```python
from build123d import *

# Parameters (mm, degrees)
BOSS_EXTRUDE1_DEPTH      = 5
BOSS_EXTRUDE2_DEPTH      = 1
BOSS_EXTRUDE2_DEPTH_BACK = 1
SKETCH4_W                = 2
SKETCH4_H                = 1
SKETCH4_W_2              = 17
SKETCH4_H_2              = 2
SKETCH5_R                = 0.75
BOSS_EXTRUDE3_DEPTH      = 5
FILLET1_R                = 4


with BuildPart() as part:
    # Sketch1 → Boss-Extrude1 (new body)
    with BuildSketch(Plane(origin=(0, 0, 0), x_dir=(1, 0, 0), z_dir=(0, 1, 0))):
        with BuildLine():
            Line((0, 14.4), (25, 14.4))
            ThreePointArc((25, 14.4), (39.4, 0), (25, -14.4))
            Line((25, -14.4), (0, -14.4))
            ThreePointArc((0, -14.4), (-14.4, 0), (0, 14.4))
        make_face()
        with BuildLine():
            Line((0, 12.4), (25, 12.4))
            ThreePointArc((25, 12.4), (37.4, 0), (25, -12.4))
            Line((25, -12.4), (0, -12.4))
            ThreePointArc((0, -12.4), (-12.4, 0), (0, 12.4))
        make_face(mode=Mode.SUBTRACT)
    extrude(amount=BOSS_EXTRUDE1_DEPTH)

    # Sketch4 → Boss-Extrude2 (add, two sides: drawn at the far end of the back side and taken through both)
    with BuildSketch(Plane.XY.offset(-BOSS_EXTRUDE2_DEPTH_BACK)):
        Polygon((-31.4, 12), (-29.4, 12), (-29.4, 13), (-32.4, 13), (-32.4, 11), (-31.4, 11), align=None)
        with Locations((-30.4, 11.5)):
            Rectangle(SKETCH4_W, SKETCH4_H)
        Polygon((-29.4, 3), (-29.4, 5), (-29.4, 11), (-31.4, 11), (-31.4, 3), align=None)
        with Locations((-20.9, 4)):
            Rectangle(SKETCH4_W_2, SKETCH4_H_2)
    extrude(amount=BOSS_EXTRUDE2_DEPTH + BOSS_EXTRUDE2_DEPTH_BACK)

    # Sketch5 → Boss-Extrude3 (add)
    with BuildSketch(Plane.ZY.offset(32.4)):
        with Locations((0, 12)):
            Circle(SKETCH5_R)
    extrude(amount=BOSS_EXTRUDE3_DEPTH)

    # Fillet1
    # the kernel refuses this fillet: 4 mm, written as the material it adds along each edge
    with BuildSketch(Plane(origin=(-14.365235814, 5, -1), x_dir=(0.17149804582148126, 0, -0.9851844600273663), z_dir=(0, -1, 0))) as fillet1_piece_1:
        with BuildLine():
            CenterArc((3.367524545, -3.978862537), FILLET1_R, 95.892851455, 74.232218513)
            Line((-0.573213295, -3.292870354), (-0.652028052, -3.27915051))
            Line((-0.652028052, -3.27915051), (-0.078814757, 0.013719844))
            Line((-0.078814757, 0.013719844), (0.008213474, 0.079577251))
            ThreePointArc((0.008213474, 0.079577251), (1.47842541, 0.003905135), (2.948637345, 0.079577251))
            Line((2.948637345, 0.079577251), (2.95685082, 0))
        make_face()
    extrude(amount=2)
    with BuildSketch(Plane(origin=(-14.365235814, 5, 1), x_dir=(0.17149804582148112, 0, 0.9851844600273663), z_dir=(0, -1, 0))) as fillet1_piece_2:
        with BuildLine():
            CenterArc((3.367524545, 3.978862537), FILLET1_R, 189.874930032, 74.232218513)
            Line((-0.573213295, 3.292870354), (-0.652028052, 3.27915051))
            Line((-0.652028052, 3.27915051), (-0.078814757, -0.013719844))
            Line((-0.078814757, -0.013719844), (0.008213474, -0.079577251))
            ThreePointArc((0.008213474, -0.079577251), (1.47842541, -0.003905135), (2.948637345, -0.079577251))
            Line((2.948637345, -0.079577251), (2.95685082, 0))
        make_face()
    extrude(amount=2)
    with BuildSketch(Plane(origin=(0, 3, 0), x_dir=(-0.7371891614816782, 0, 0.6756864214959037), z_dir=(0.6756864214959037, 0, 0.7371891614816782))) as fillet1_piece_3_section:
        with BuildLine():
            CenterArc((18.272983346, 4), FILLET1_R, 194.477512186, 75.522487814)
            Line((18.272983346, 0), (18.272983346, -0.08))
            Line((18.272983346, -0.08), (14.4, -0.08))
            Line((14.4, -0.08), (14.32, 0))
            ThreePointArc((14.32, 0), (14.32, 1.5), (14.322540333, 2.98))
            Line((14.322540333, 2.98), (14.4, 3))
        make_face()
    fillet1_piece_3 = revolve(axis=Axis((0, 3, 0), (0, -1, 0)), revolution_arc=85.014954966, mode=Mode.PRIVATE)
    fillet1_piece_3 = split(fillet1_piece_3, bisect_by=Plane(origin=(-15.301586286, 2.241601932, -1), z_dir=(0, 0, 1)), keep=Keep.TOP, mode=Mode.PRIVATE)
    fillet1_piece_3 = split(fillet1_piece_3, bisect_by=Plane(origin=(-15.301586286, 2.241601932, 1), z_dir=(0, 0, -1)), keep=Keep.TOP, mode=Mode.PRIVATE)
    add(fillet1_piece_3)
    with BuildSketch(Plane(origin=(-29.4, 5, 1), x_dir=(1, 0, 0), z_dir=(0, 0, -1))) as fillet1_piece_4:
        with BuildLine():
            CenterArc((FILLET1_R, -FILLET1_R), FILLET1_R, 90, 90)
            Line((0, -FILLET1_R), (-FILLET1_R * 0.02, -FILLET1_R))
            Line((-FILLET1_R * 0.02, -FILLET1_R), (-FILLET1_R * 0.02, FILLET1_R * 0.02))
            Line((-FILLET1_R * 0.02, FILLET1_R * 0.02), (FILLET1_R, FILLET1_R * 0.02))
            Line((FILLET1_R, FILLET1_R * 0.02), (FILLET1_R, 0))
        make_face()
    extrude(amount=2)
    with BuildSketch(Plane(origin=(-31.4, 11, -1), x_dir=(0, -1, 0), z_dir=(0, 0, 1))) as fillet1_piece_5:
        with BuildLine():
            CenterArc((2.645751311, -4), FILLET1_R, 90, 41.409622109)
            Line((0, -1), (-0.052915026, -0.94))
            ThreePointArc((-0.052915026, -0.94), (-0.08, -0.5), (-0.08, 0))
            Line((-0.08, 0), (0, 0.08))
            Line((0, 0.08), (2.645751311, 0.08))
            Line((2.645751311, 0.08), (2.645751311, 0))
        make_face()
    extrude(amount=2)
    with BuildSketch(Plane(origin=(-14.365235814, 5, -1), x_dir=(0.17149804582148126, 0, -0.9851844600273663), z_dir=(0, -1, 0))) as fillet1_piece_6a_section:
        with BuildLine():
            CenterArc((3.367524545, -3.978862537), FILLET1_R, 95.892851455, 74.232218513)
            Line((-0.573213295, -3.292870354), (-0.652028052, -3.27915051))
            Line((-0.652028052, -3.27915051), (-0.078814757, 0.013719844))
            Line((-0.078814757, 0.013719844), (0.008213474, 0.079577251))
            ThreePointArc((0.008213474, 0.079577251), (1.47842541, 0.003905135), (2.948637345, 0.079577251))
            Line((2.948637345, 0.079577251), (2.95685082, 0))
        make_face()
    fillet1_piece_6a = extrude(amount=10.355974154, mode=Mode.PRIVATE)
    fillet1_piece_6a = split(fillet1_piece_6a, bisect_by=Plane(origin=(-15.057221624, 0, -1.646357347), z_dir=(0, 1, 0)), keep=Keep.TOP, mode=Mode.PRIVATE)
    fillet1_piece_6a = split(fillet1_piece_6a, bisect_by=Plane(origin=(-15.057221624, 3, -1.646357347), z_dir=(0, -1, 0)), keep=Keep.TOP, mode=Mode.PRIVATE)
    with BuildSketch(Plane(origin=(0, 3, 0), x_dir=(-0.7371891614816782, 0, 0.6756864214959037), z_dir=(0.6756864214959037, 0, 0.7371891614816782))) as fillet1_piece_6b_section:
        with BuildLine():
            CenterArc((18.272983346, 4), FILLET1_R, 194.477512186, 75.522487814)
            Line((18.272983346, 0), (18.272983346, -0.08))
            Line((18.272983346, -0.08), (14.4, -0.08))
            Line((14.4, -0.08), (14.32, 0))
            ThreePointArc((14.32, 0), (14.32, 1.5), (14.322540333, 2.98))
            Line((14.322540333, 2.98), (14.4, 3))
        make_face()
    fillet1_piece_6b = revolve(axis=Axis((0, 3, 0), (0, -1, 0)), revolution_arc=85.014954966, mode=Mode.PRIVATE)
    fillet1_piece_6b = split(fillet1_piece_6b, bisect_by=Plane(origin=(-13.861423807, 2.266551545, -1), z_dir=(0, 0, -1)), keep=Keep.TOP, mode=Mode.PRIVATE)
    fillet1_piece_6 = fillet1_piece_6a & fillet1_piece_6b
    add(fillet1_piece_6)
    with BuildSketch(Plane(origin=(0, 3, 0), x_dir=(-0.7371891614816782, 0, 0.6756864214959037), z_dir=(0.6756864214959037, 0, 0.7371891614816782))) as fillet1_piece_7a_section:
        with BuildLine():
            CenterArc((18.272983346, 4), FILLET1_R, 194.477512186, 75.522487814)
            Line((18.272983346, 0), (18.272983346, -0.08))
            Line((18.272983346, -0.08), (14.4, -0.08))
            Line((14.4, -0.08), (14.32, 0))
            ThreePointArc((14.32, 0), (14.32, 1.5), (14.322540333, 2.98))
            Line((14.322540333, 2.98), (14.4, 3))
        make_face()
    fillet1_piece_7a = revolve(axis=Axis((0, 3, 0), (0, -1, 0)), revolution_arc=85.014954966, mode=Mode.PRIVATE)
    fillet1_piece_7a = split(fillet1_piece_7a, bisect_by=Plane(origin=(-13.861424305, 2.266551683, 1), z_dir=(0, 0, 1)), keep=Keep.TOP, mode=Mode.PRIVATE)
    with BuildSketch(Plane(origin=(-14.365235814, 5, 1), x_dir=(0.17149804582148112, 0, 0.9851844600273663), z_dir=(0, -1, 0))) as fillet1_piece_7b_section:
        with BuildLine():
            CenterArc((3.367524545, 3.978862537), FILLET1_R, 189.874930032, 74.232218513)
            Line((-0.573213295, 3.292870354), (-0.652028052, 3.27915051))
            Line((-0.652028052, 3.27915051), (-0.078814757, -0.013719844))
            Line((-0.078814757, -0.013719844), (0.008213474, -0.079577251))
            ThreePointArc((0.008213474, -0.079577251), (1.47842541, -0.003905135), (2.948637345, -0.079577251))
            Line((2.948637345, -0.079577251), (2.95685082, 0))
        make_face()
    fillet1_piece_7b = extrude(amount=10.355974154, mode=Mode.PRIVATE)
    fillet1_piece_7b = split(fillet1_piece_7b, bisect_by=Plane(origin=(-15.057221624, 0, 1.646357347), z_dir=(0, 1, 0)), keep=Keep.TOP, mode=Mode.PRIVATE)
    fillet1_piece_7b = split(fillet1_piece_7b, bisect_by=Plane(origin=(-15.057221624, 3, 1.646357347), z_dir=(0, -1, 0)), keep=Keep.TOP, mode=Mode.PRIVATE)
    fillet1_piece_7 = fillet1_piece_7a & fillet1_piece_7b
    add(fillet1_piece_7)
    # the kernel refuses this fillet: 4 mm, written as the material it takes off along each edge
    with BuildSketch(Plane(origin=(-31.4, 3, -11), x_dir=(1, 0, 0), z_dir=(0, 0, 1))) as fillet1_2_piece_1:
        with BuildLine():
            CenterArc((FILLET1_R, FILLET1_R), FILLET1_R, 180, 90)
            Line((0, FILLET1_R), (-FILLET1_R * 0.02, FILLET1_R))
            Line((-FILLET1_R * 0.02, FILLET1_R), (-FILLET1_R * 0.02, -FILLET1_R * 0.02))
            Line((-FILLET1_R * 0.02, -FILLET1_R * 0.02), (FILLET1_R, -FILLET1_R * 0.02))
            Line((FILLET1_R, -FILLET1_R * 0.02), (FILLET1_R, 0))
        make_face()
    extrude(amount=22, mode=Mode.SUBTRACT)
    with BuildSketch(Plane(origin=(-29.4, 13, -10.682458366), x_dir=(-1, 0, 0), z_dir=(0, 0, 1))) as fillet1_2_piece_2:
        with BuildLine():
            CenterArc((4, 3.872983346), FILLET1_R, 180, 75.522487814)
            Line((0, 3.872983346), (-0.08, 3.872983346))
            Line((-0.08, 3.872983346), (-0.08, 0))
            Line((-0.08, 0), (0, -0.08))
            ThreePointArc((0, -0.08), (1.5, -0.08), (2.98, -0.077459667))
            Line((2.98, -0.077459667), (3, 0))
        make_face()
    extrude(amount=21.364916731, mode=Mode.SUBTRACT)


solid = part.part
```
Part model, mm, in its own coordinate system. A direction names the side the tool comes from. Give positions to 0.01 mm unless a question says otherwise; leave off trailing zeros. Order: outer loops, then holes, each group sorted by start corner. A loop starts at its lowest first (then second) coordinate and runs counter-clockwise, first axis right, second up. Notation, with made-up numbers: (70, 39.25) - (108, 39.25) arc R27 ccw to (108, 77.25) - close; hole circle Ø9 at (80.5, 62.5). An arc over 180 degrees is marked (long way). Use one line per item in the form item = value.
Item 1: Slice it at B-B on x = -11.5. Give the cut face in (y, z), and give its area (3 significant figures).
Solution:
outline = (0, -8.67) - (5, -8.67) - (5, -4.64) - (0, -4.64) - close; (0, 4.64) - (5, 4.64) - (5, 8.67) - (0, 8.67) - close
area = 40.3 mm2
Item 2: Pin check, flat tips, straight feed: pin 1 Ø1 at (x, y) = (26, 2.5) entering from +Z; pin 2 Ø2 at (x, z) = (-24.5, 0.5) entering from -Y; pin 3 Ø3 at (x, y) = (-11, 4.5) entering from -Z. Stop position of each tip, or through.
Solution:
pin_1 = 14.39
pin_2 = 3
pin_3 = -10.82
Item 3: Slice it at D-D on y = 12. Give the cut face in (x, z), and give its area (3 significant figures).
Solution:
outline = (-37.4, -0.75) - (-32.4, -0.75) - (-32.4, -1) - (-30.62, -1) - (-30.62, 1) - (-32.4, 1) - (-32.4, 0.75) - (-37.4, 0.75) - close
area = 11.1 mm2
Item 4: Slice it at A-A on z = 0. Give the cut face in (x, y).
Solution:
outline = (-37.4, 11.25) - (-32.4, 11.25) - (-32.4, 11) arc R4 cw to (-31.4, 8.35) - (-31.4, 7) arc R4 ccw to (-27.4, 3) - (-18.27, 3) arc R4 cw to (-14.4, 0) - (-12.4, 0) - (-12.4, 5) - (-25.4, 5) arc R4 cw to (-29.4, 9) - (-29.4, 9.13) arc R4 ccw to (-32.4, 13) - (-32.4, 12.75) - (-37.4, 12.75) - close; (37.4, 0) - (39.4, 0) - (39.4, 5) - (37.4, 5) - close
Item 5: Two-plate mould, pull along X, no slides. Class faces 5 (the face through (13, 0, 13)), 6 (the face through (39.397, 2.465, -0.317)), 7 (the face through (37.397, 2.465, -0.273)): released by +X, released by -X, zero draft, split by the parting line, or undercut.
Solution:
face_5 = zero draft
face_6 = released by +X
face_7 = undercut
Item 6: Probe probe 1 along Z at (x, y) = (10, 4.25); probe 2 along Z at (x, y) = (-29, 3.5); probe 3 along X at (y, z) = (1.5, 10). List the from-to ranges inside material, lowest first. Write a range as from..to.
Solution:
probe_1 = -14.4..-12.4, 12.4..14.4
probe_2 = -1..1
probe_3 = -10.36..-7.33, 32.33..35.36
Item 7: Slice it at C-C on y = 2. Give the cut face in (x, z), and give its area (3 significant figures).
Solution:
outline = (-15.54, -1.64) arc R4 cw to (-13.86, -3.91) arc R14.4 ccw to (0, -14.4) - (25, -14.4) arc R14.4 ccw to (25, 14.4) - (0, 14.4) arc R14.4 ccw to (-13.86, 3.91) arc R4 cw to (-15.54, 1.64) arc R15.63 ccw to start; hole (0, -12.4) - (25, -12.4) arc R12.4 ccw to (25, 12.4) - (0, 12.4) arc R12.4 ccw to start
area = 274 mm2
Item 8: Which spindle directions (+Z, -Z, +X, -X, +Y, -Y) get a long thin tool onto all of the face, cutting with end or side? Do faces 1 (the face through (-27, 5, 1)), 2 (the face through (-31.4, 8, 0)), 3 (the face through (-34.865, 12.744, -0.098)), 4 (the face through (12, 2, -12.4)). Say none if no direction does.
Solution:
face_1 = +Z, -X, +Y, -Y
face_2 = +Z, -Z, -X, -Y
face_3 = -X
face_4 = +Y, -Y
